Geometry: see drawing. Coordinates: mm, zero at the bounding-box minimum. A direction names the side the tool comes from. Coordinates: 2 decimals unless noted, no trailing zeros. Loops run counter-clockwise (first coordinate to the right, second up) from the corner with the lowest first, then second, coordinate; pieces in that order, holes last. Notation, with made-up numbers: M 13,47.25 L 33,47.25 A29 ccw 33,75.25 Z; hole C -21,85.5 d1. An arc over 180 degrees is marked long. Write each question's results on one line, items separated by ' | '. Start each with the question number.
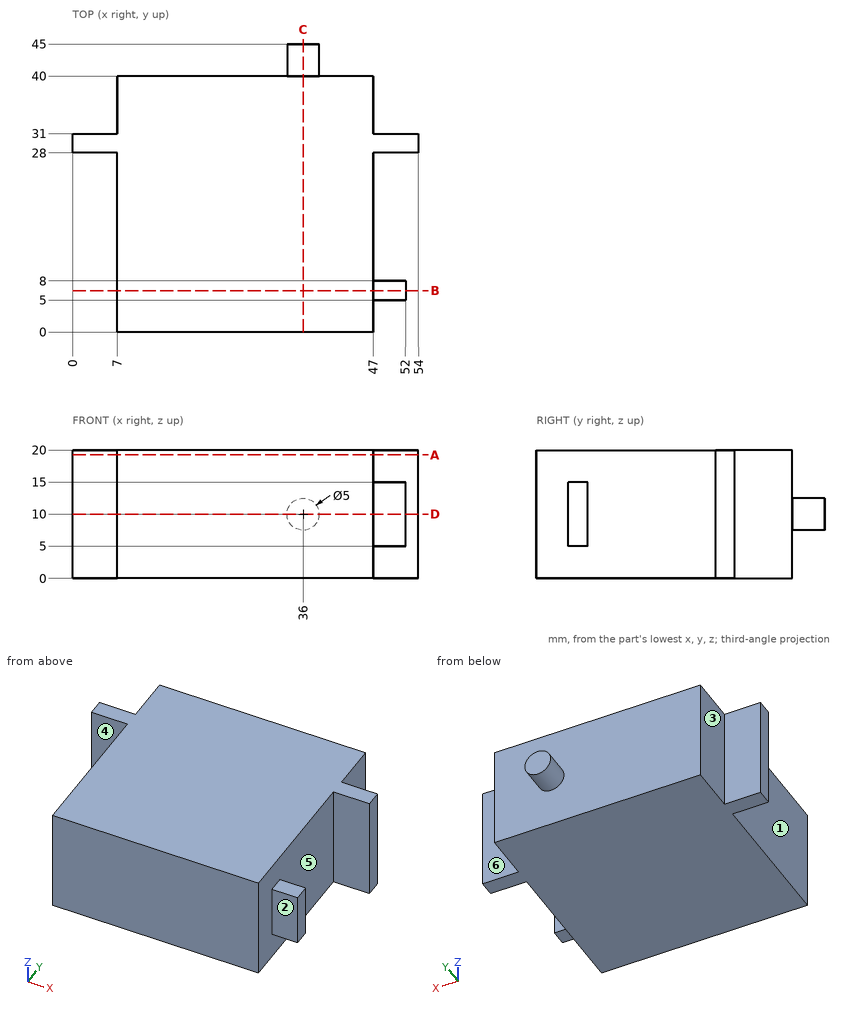
Item 1: Mould query, pull axis Y, two halves, no side actions, for the marked faces 4, 5 and 6. Classes: +Y half, -Y half, draft (parallel to the pull), parting line (faces both ways), or undercut.
Item 2: Cut plane C-C (x = 36). Output: boundary loops of the cut face in (y, z), then the cut area to 3 significant figures.
Item 3: First-contact query: pin 1 Ø5 at (x, y) = (13.5, 35) entering from -Z; pin 2 Ø3.5 at (x, y) = (50, 6.5) entering from +Z; pin 3 Ø5 at (y, z) = (19.5, 15.5) entering from +X; pin 4 Ø3.5 at (x, z) = (51, 5) entering from +Y. Flat tips, straight axial feed; report the tip coordinate or a pass-through.
Item 4: Cut plane B-B (y = 6.5). Output: boundary loops of the cut face in (x, z), then the cut area to 3 significant figures.
Item 5: Line query: probe 1 along Y at (x, z) = (49, 14); probe 2 along Y at (x, z) = (32, 8); probe 3 along X at (y, z) = (36.5, 14.25). Output: solid intervals per line, ascending.
Item 6: Cut plane A-A (z = 19.25). Output: boundary loops of the cut face in (x, y), then the cut area to 3 significant figures.
Item 7: Cut plane D-D (z = 10). Output: boundary loops of the cut face in (x, y).
Item 8: Access query for the marked faces 1, 2 and 3. Directions: +Z, -Z, +X, -X, +Y, -Y. A direction counts if a zero-diameter tool reaches every point of the face in a straight line with its end or side. Return the directions, or none.
Response values:
1) face 4: -Y half | face 5: undercut | face 6: +Y half
2) outline: M 0,0 L 40,0 L 40,7.5 L 45,7.5 L 45,12.5 L 40,12.5 L 40,20 L 0,20 Z | area: 825 mm2
3) pin 1: stops at z = 0 | pin 2: stops at z = 15 | pin 3: stops at x = 47 | pin 4: stops at y = 31
4) outline: M 7,0 L 47,0 L 47,5 L 52,5 L 52,15 L 47,15 L 47,20 L 7,20 Z | area: 850 mm2
5) probe 1: y = 5 to 8, 28 to 31 | probe 2: y = 0 to 40 | probe 3: x = 7 to 47
6) outline: M 0,28 L 7,28 L 7,0 L 47,0 L 47,28 L 54,28 L 54,31 L 47,31 L 47,40 L 7,40 L 7,31 L 0,31 Z | area: 1,640 mm2
7) outline: M 0,28 L 7,28 L 7,0 L 47,0 L 47,5 L 52,5 L 52,8 L 47,8 L 47,28 L 54,28 L 54,31 L 47,31 L 47,40 L 38.5,40 L 38.5,45 L 33.5,45 L 33.5,40 L 7,40 L 7,31 L 0,31 Z
8) face 1: +Z, -Z, -X, -Y | face 2: +Z, -Z, +X, -Y | face 3: +Z, -Z, -X, +Y
